```python
from build123d import *

# Parameters (mm, degrees)
F1_DEPTH       = 10
F3_D           = 5.8
F3_CBORE_D     = 9.75
F3_CBORE_DEPTH = 5
F4_R           = 3.3399169876
F5_DEPTH       = 25
F6_D           = 3.6
F6_CBORE_D     = 6.5
F6_CBORE_DEPTH = 3
F7_W           = 3
F7_H           = 6
F8_DEPTH       = 7
F9_R           = 1


with BuildPart() as f1:
    # F0 (on Top) → F1 (new body)
    with BuildSketch(Plane.XY):
        with BuildLine():
            Line((-15, 12.5), (-15, -12.5))
            Line((-15, -12.5), (15, -12.5))
            Line((15, -12.5), (15, 11.6508761421))
            Line((15, 11.6508761421), (8.2564513366, 11.6508761421))
            ThreePointArc((8.2564513366, 11.6508761421), (-8.2998116615, 12.5559140775), (8.2671421606, 13.2378078997))
            Line((8.2671421606, 13.2378078997), (14.9818436617, 13.2378078997))
            Line((14.9818436617, 13.2378078997), (14.9818436617, 20.172925666))
            Line((14.9818436617, 20.172925666), (12.8889957609, 20.172925666))
            ThreePointArc((12.8889957609, 20.172925666), (-3.979011409, 26.962623144), (-15, 12.5))
        make_face()
    extrude(amount=F1_DEPTH)

    # F3 (through all)
    with Locations(Plane(origin=(0, 0, 0), x_dir=(1, 0, 0), z_dir=(0, 0, -1))):
        with Locations((0, 4.9573802389)):
            CounterBoreHole(F3_D / 2, F3_CBORE_D / 2, F3_CBORE_DEPTH)

    # F4 (on face) → F5 (cut)
    with BuildSketch(Plane(origin=(0, 20.172925666, 0), x_dir=(-1, 0, 0), z_dir=(0, 1, 0))):
        with Locations((-11.4818436617, 5)):
            Circle(F4_R)
    extrude(amount=F5_DEPTH, mode=Mode.SUBTRACT)

    # F6 (through all)
    with Locations(Plane(origin=(0, 20.172925666, 0), x_dir=(-1, 0, 0), z_dir=(0, 1, 0))):
        with Locations((-11.4818436617, 5)):
            CounterBoreHole(F6_D / 2, F6_CBORE_D / 2, F6_CBORE_DEPTH)

    # F7 (on face) → F8 (cut)
    with BuildSketch(Plane.YZ.offset(15)):
        with Locations((4.0933839045, 5)):
            Rectangle(F7_W, F7_H)
    extrude(amount=-F8_DEPTH, mode=Mode.SUBTRACT)

    # F9
    f9_edges = [f1.edges().sort_by_distance(p)[0] for p in [
        (-8.299812, 12.555914, 0),
    ]]
    fillet(f9_edges, radius=F9_R)


solid = f1.part
```
For this review, take the finished solid that the model builds, in its own axes (mm). A direction names the side the tool comes from. Coordinates: 2 decimals unless noted, no trailing zeros. Loops run counter-clockwise (first coordinate to the right, second up) from the corner with the lowest first, then second, coordinate; pieces in that order, holes last. Notation, with made-up numbers: (40.25, -34) - (97.25, -34) arc R17 cw to (97.25, -9) - close; hole circle Ø11 at (52.5, 3.5). An arc over 180 degrees is marked (long way). Use one line per item in the form item = value. Start each with the question number.
1) For faces 4 (the face through (13.2, 11.651, 3.8)), 5 (the face through (8.143, 22.054, 4.906)), 6 (the face through (12, 4, 2)), list the 3-axis set-ups (+Z, -Z, +X, -X, +Y, -Y) from which the entire face can be reached by the end or side of a thin tool; tool diameter is ignored.
2) Take a section at B-B (y = -2.5). State the section outline as (x, z) points.
3) Take a section at A-A (x = 11.5). State how many separate pieces and enclosed holes the cut face has, plus the area to 3 significant figures.
4) Draft analysis for pull direction Z (two halves, no side actions). For faces 1 (the face through (15, -1, 5)), 2 (the face through (-4, 3, 0)), 3 (the face through (10.053, 15.178, 3.905)), state which applies: released by +Z, released by -Z, zero draft, split by the parting line, or undercut.
5) For pin 1 (5 mm diameter, centred on x = -1.5, y = -3.5, fed in from -Z); pin 2 (1.5 mm diameter, centred on x = -3.5, y = 5.5, fed in from -Z); pin 3 (4 mm diameter, centred on x = -4, z = 5.5, fed in from +Y); pin 4 (3 mm diameter, centred on x = 11.48, z = 5, fed in from -Y) (3 decimals), all flat-tipped, find the tip position at first contact; note any pin that passes through.
6) To check wall thickness, follow probe 1 along Y at (x, z) = (12, 7.5); probe 2 along Y at (x, z) = (12.5, 8.5); probe 3 along Z at (x, y) = (10.5, 3.5). State the ranges of each line that lie inside material, in increasing order. Write a range as from..to.
From the geometry:
q1.face_4 = +Z, -Z, +X
q1.face_5 = +Y
q1.face_6 = +X
q2.outline = (-15, 0) - (-4.21, 0) - (-4.21, 5) - (-1.54, 5) - (-1.54, 10) - (-15, 10) - close; (1.54, 5) - (4.21, 5) - (4.21, 0) - (15, 0) - (15, 10) - (1.54, 10) - close; hole circle Ø3.6 at (11.48, 5)
q3.separate_pieces = 4
q3.enclosed_holes = 0
q3.area = 190 mm2
q4.face_1 = zero draft
q4.face_2 = released by -Z
q4.face_3 = undercut
q5.pin_1 = 5
q5.pin_2 = 0.31
q5.pin_3 = 27.37
q5.pin_4 = through
q6.probe_1 = -12.5..2.59, 5.59..11.65, 13.24..17.17
q6.probe_2 = -12.5..11.65, 13.24..20.79
q6.probe_3 = 0..2, 8..10
